```python
from build123d import *

# Parameters (mm, degrees)
SKETCH1_R             = 12.5
BOSS_EXTRUDE1_DEPTH   = 20
SKETCH2_R             = 10
BOSS_EXTRUDE2_DEPTH   = 2
LPATTERN4_START       = 22
LPATTERN4_OUTLINE_R   = 12.5
LPATTERN4_DEPTH       = 20
LPATTERN4_START_2     = -2
LPATTERN4_2_OUTLINE_R = 10
LPATTERN4_2_DEPTH     = 46
LPATTERN5_COUNT       = 5
LPATTERN5_PITCH       = 22


# Read off the part's stored shape, not the designer's step: LPattern4
with BuildPart() as part:
    # Sketch1 → Boss-Extrude1 (new body)
    with BuildSketch(Plane(origin=(0, 0, 0), x_dir=(0, 0, -1), z_dir=(1, 0, 0))):
        Circle(SKETCH1_R)
    boss_extrude1 = extrude(amount=BOSS_EXTRUDE1_DEPTH)

    # Sketch2 → Boss-Extrude2 (add)
    with BuildSketch(Plane(origin=(20, 0, 0), x_dir=(0, 0, -1), z_dir=(1, 0, 0))):
        Circle(SKETCH2_R)
    extrude(amount=BOSS_EXTRUDE2_DEPTH)

    # LPattern4 outline → LPattern4 (add)
    with BuildSketch(Plane.YZ.offset(LPATTERN4_START)):
        Circle(LPATTERN4_OUTLINE_R)
    lpattern4 = extrude(amount=LPATTERN4_DEPTH)

    # LPattern4 2 outline → LPattern4 2 (add)
    with BuildSketch(Plane.YZ.offset(LPATTERN4_START_2)):
        Circle(LPATTERN4_2_OUTLINE_R)
    lpattern4_2 = extrude(amount=LPATTERN4_2_DEPTH)

    # LPattern5: Boss-Extrude1, LPattern4, LPattern4 2 ×5
    with Locations(*[(-i * LPATTERN5_PITCH, 0, 0) for i in range(1, LPATTERN5_COUNT)]):
        add(boss_extrude1)
        add(lpattern4)
        add(lpattern4_2)


solid = part.part
```
Geometry check sheet. Reference: the model listing, model coordinates, mm. A direction names the side the tool comes from. Round coordinates to 2 decimals unless told otherwise and drop trailing zeros. Order: outer loops, then holes, each group sorted by start corner. A loop starts at its lowest first (then second) coordinate and runs counter-clockwise, first axis right, second up. Notation, with made-up numbers: (-28.75, 23.25) - (-4.75, 23.25) arc R20 ccw to (-4.75, 44.25) - close; hole circle Ø5 at (1.25, 5). An arc over 180 degrees is marked (long way). Use a Markdown table: item, result. Add a question column.
(1) Tool access check on faces 1 (the flat face through (-66, 10.2, 0.1)), 2 (the cylindrical face through (42.99, -2.17, -9.76)), 3 (the flat face through (-88, 10.2, 0.1)), 4 (the cylindrical face through (-34.14, 3.755, -11.923)). Record the directions out of +Z, -Z, +X, -X, +Y, -Y that give a thin tool (end or side, any length) a straight path to the whole face; none if there is none.
(2) Release check for a two-part mould opening along X. For faces 5 (the cylindrical face through (-89.01, -2.17, -9.76)), 6 (the cylindrical face through (-1.01, -2.17, -9.76)), 7 (the flat face through (-90, 0, 0)) record: pulls with the +X half, pulls with the -X half, needs draft (parallel to the pull), parting line crosses it, or undercut.
(3) Depth check by flat-ended pin: pin 1 (12 mm diameter, centred on x = -62.5, y = -9, fed in from -Z); pin 2 (3 mm diameter, centred on x = -63, z = 8, fed in from -Y); pin 3 (8 mm diameter, centred on x = -34.5, y = 4.5, fed in from -Z). Enter the tip coordinate at first touch or a pass-through.
(4) Sectioned sample at A-A, the plane x = 6. Enter the section's corners in (y, z).
(5) Material ranges on line 1 along X through (y, z) = (-6, 9.75); line 2 along Z through (x, y) = (26, 0); line 3 along Z through (x, y) = (-80.5, 8), recorded low to high. Write a range as [from, to].
Answers below:
| question | item | result |
|---|---|---|
| 1 | face 1 | none |
| 1 | face 2 | +X |
| 1 | face 3 | -X |
| 1 | face 4 | +X, -X |
| 2 | face 5 | needs draft |
| 2 | face 6 | undercut |
| 2 | face 7 | pulls with the -X half |
| 3 | pin 1 | z = -12.13 |
| 3 | pin 2 | y = -10.68 |
| 3 | pin 3 | z = -12.49 |
| 4 | outline | circle Ø25 at (0, 0) |
| 5 | line 1 | [-88, -68], [-66, -46], [-44, -24], [-22, -2], [0, 20], [22, 42] |
| 5 | line 2 | [-12.5, 12.5] |
| 5 | line 3 | [-9.6, 9.6] |
